from build123d import *

# Parameters (mm, degrees)
SKETCH1_W                 = 50.8889
SKETCH1_H                 = 6.35
BOSS_EXTRUDE1_DEPTH       = 225.99904
SKETCH3_R                 = 5.000000033
CUT_EXTRUDE1_DEPTH        = 228.515512914
LPATTERN1_COUNT           = 3
LPATTERN1_PITCH           = 11.500000114
LPATTERN1_COUNT_DIR2      = 3
LPATTERN1_PITCH_DIR2      = 11.500000114
LPATTERN2_COUNT           = 2
LPATTERN2_PITCH           = 66.00000008
LPATTERN2_COPY_1_SKETCH_R = 5.000000033
LPATTERN2_COPY_1_DEPTH    = 228.515512914
LPATTERN2_COPY_2_SKETCH_R = 5.000000033
LPATTERN2_COPY_2_DEPTH    = 228.515512914
LPATTERN2_COPY_3_SKETCH_R = 5.000000033
LPATTERN2_COPY_3_DEPTH    = 228.515512914
LPATTERN2_COPY_4_SKETCH_R = 5.000000033
LPATTERN2_COPY_4_DEPTH    = 228.515512914
LPATTERN2_COPY_5_SKETCH_R = 5.000000033
LPATTERN2_COPY_5_DEPTH    = 228.515512914
LPATTERN2_COPY_6_SKETCH_R = 5.000000033
LPATTERN2_COPY_6_DEPTH    = 228.515512914
LPATTERN2_COPY_7_SKETCH_R = 5.000000033
LPATTERN2_COPY_7_DEPTH    = 228.515512914
LPATTERN2_COPY_8_SKETCH_R = 5.000000033
LPATTERN2_COPY_8_DEPTH    = 228.515512914


with BuildPart() as part:
    # Sketch1 → Boss-Extrude1 (new body)
    with BuildSketch(Plane.XY):
        Rectangle(SKETCH1_W, SKETCH1_H)
    extrude(amount=BOSS_EXTRUDE1_DEPTH)

    # Sketch3 → Cut-Extrude1 (cut, through all)
    with BuildSketch(Plane(origin=(0, 3.175, 0), x_dir=(1, 0, 0), z_dir=(0, 1, 0))):
        with Locations(Location((8.669450022, -180.875882939, 0), (0, 0, 270))):
            Circle(SKETCH3_R)
    cut_extrude1 = extrude(amount=-CUT_EXTRUDE1_DEPTH, mode=Mode.SUBTRACT)

    # LPattern1: Cut-Extrude1 3 × 3
    with Locations(*[(-i * LPATTERN1_PITCH, 0, -j * LPATTERN1_PITCH_DIR2) for i in range(LPATTERN1_COUNT) for j in range(LPATTERN1_COUNT_DIR2) if (i, j) != (0, 0)]):
        add(cut_extrude1, mode=Mode.SUBTRACT)

    # LPattern2: Cut-Extrude1 ×2
    with Locations(*[(0, 0, -i * LPATTERN2_PITCH) for i in range(1, LPATTERN2_COUNT)]):
        add(cut_extrude1, mode=Mode.SUBTRACT)

    # LPattern2 copy 1 sketch → LPattern2 copy 1 (cut, through all)
    with BuildSketch(Plane(origin=(0, 3.175, -77.500000194), x_dir=(1, 0, 0), z_dir=(0, 1, 0))):
        with Locations(Location((8.669450022, -180.875882939, 0), (0, 0, 270))):
            Circle(LPATTERN2_COPY_1_SKETCH_R)
    extrude(amount=-LPATTERN2_COPY_1_DEPTH, mode=Mode.SUBTRACT)

    # LPattern2 copy 2 sketch → LPattern2 copy 2 (cut, through all)
    with BuildSketch(Plane(origin=(0, 3.175, -89.000000308), x_dir=(1, 0, 0), z_dir=(0, 1, 0))):
        with Locations(Location((8.669450022, -180.875882939, 0), (0, 0, 270))):
            Circle(LPATTERN2_COPY_2_SKETCH_R)
    extrude(amount=-LPATTERN2_COPY_2_DEPTH, mode=Mode.SUBTRACT)

    # LPattern2 copy 3 sketch → LPattern2 copy 3 (cut, through all)
    with BuildSketch(Plane(origin=(-11.500000114, 3.175, -66.00000008), x_dir=(1, 0, 0), z_dir=(0, 1, 0))):
        with Locations(Location((8.669450022, -180.875882939, 0), (0, 0, 270))):
            Circle(LPATTERN2_COPY_3_SKETCH_R)
    extrude(amount=-LPATTERN2_COPY_3_DEPTH, mode=Mode.SUBTRACT)

    # LPattern2 copy 4 sketch → LPattern2 copy 4 (cut, through all)
    with BuildSketch(Plane(origin=(-11.500000114, 3.175, -77.500000194), x_dir=(1, 0, 0), z_dir=(0, 1, 0))):
        with Locations(Location((8.669450022, -180.875882939, 0), (0, 0, 270))):
            Circle(LPATTERN2_COPY_4_SKETCH_R)
    extrude(amount=-LPATTERN2_COPY_4_DEPTH, mode=Mode.SUBTRACT)

    # LPattern2 copy 5 sketch → LPattern2 copy 5 (cut, through all)
    with BuildSketch(Plane(origin=(-11.500000114, 3.175, -89.000000308), x_dir=(1, 0, 0), z_dir=(0, 1, 0))):
        with Locations(Location((8.669450022, -180.875882939, 0), (0, 0, 270))):
            Circle(LPATTERN2_COPY_5_SKETCH_R)
    extrude(amount=-LPATTERN2_COPY_5_DEPTH, mode=Mode.SUBTRACT)

    # LPattern2 copy 6 sketch → LPattern2 copy 6 (cut, through all)
    with BuildSketch(Plane(origin=(-23.000000228, 3.175, -66.00000008), x_dir=(1, 0, 0), z_dir=(0, 1, 0))):
        with Locations(Location((8.669450022, -180.875882939, 0), (0, 0, 270))):
            Circle(LPATTERN2_COPY_6_SKETCH_R)
    extrude(amount=-LPATTERN2_COPY_6_DEPTH, mode=Mode.SUBTRACT)

    # LPattern2 copy 7 sketch → LPattern2 copy 7 (cut, through all)
    with BuildSketch(Plane(origin=(-23.000000228, 3.175, -77.500000194), x_dir=(1, 0, 0), z_dir=(0, 1, 0))):
        with Locations(Location((8.669450022, -180.875882939, 0), (0, 0, 270))):
            Circle(LPATTERN2_COPY_7_SKETCH_R)
    extrude(amount=-LPATTERN2_COPY_7_DEPTH, mode=Mode.SUBTRACT)

    # LPattern2 copy 8 sketch → LPattern2 copy 8 (cut, through all)
    with BuildSketch(Plane(origin=(-23.000000228, 3.175, -89.000000308), x_dir=(1, 0, 0), z_dir=(0, 1, 0))):
        with Locations(Location((8.669450022, -180.875882939, 0), (0, 0, 270))):
            Circle(LPATTERN2_COPY_8_SKETCH_R)
    extrude(amount=-LPATTERN2_COPY_8_DEPTH, mode=Mode.SUBTRACT)


solid = part.part
Design review of the part built by this model. Coordinates are the model's own, in mm. Give positions to 0.01 mm unless a question says otherwise; leave off trailing zeros. Write each loop counter-clockwise with the first axis right and the second up, starting at its lowest first coordinate (ties: lowest second). Pieces come first, ordered by that corner, then holes. Notation, with made-up numbers: M -20.75,-30.75 L 10.25,-30.75 A20 cw 10.25,-4.75 Z; hole C 56,84 d1. An arc over 180 degrees is marked long. Return JSON: item names as keys, results as strings. Group by question number.
Item 1: Take a section at B-B (x = 11). Give the boundary of the cut face in (y, z) (3 decimals), plus the area to 3 significant figures.
Item 2: Wall thickness on line 1 along X through (y, z) = (-2.5, 158); line 2 along X through (y, z) = (1, 93.5): over which ranges is each line inside the solid? List them lowest first.
Item 3: Take a section at C-C (y = -1.75). Count the separate pieces of the cut face and the enclosed holes in it, plus the area to 3 significant figures.
Item 4: Take a section at A-A (z = 89). Give the boundary of the cut face in (x, y) (3 decimals), plus the area to 3 significant figures.
Item 5: Clearance check with a flat-ended pin moving along its axis: pin 1 Ø6 at (x, z) = (8.67, 180.88) entering from -Y. State where the tip first meets the part, or that it passes through.
Item 6: The part is to be moulded in two halves that separate along X. For faces 1 (the cylindrical face through (-4.746, 0.044, 173.995)), 2 (the flat face through (25.444, 0, 111)), 3 (the flat face through (17, 3.175, 111)), 4 (the cylindrical face through (-14.11, 0.04, 109.88)), say which applies: pulls with the +X half, pulls with the -X half, needs draft (parallel to the pull), parting line crosses it, or undercut.
Item 7: Take a section at D-D (x = -5.5). Give the boundary of the cut face in (y, z) (3 decimals).
Return value:
{
 "1": {"outline": "M -3.175,0 L 3.175,0 L 3.175,87.452 L -3.175,87.452 Z; M -3.175,96.3 L 3.175,96.3 L 3.175,98.952 L -3.175,98.952 Z; M -3.175,107.8 L 3.175,107.8 L 3.175,110.452 L -3.175,110.452 Z; M -3.175,119.3 L 3.175,119.3 L 3.175,153.452 L -3.175,153.452 Z; M -3.175,162.3 L 3.175,162.3 L 3.175,164.952 L -3.175,164.952 Z; M -3.175,173.8 L 3.175,173.8 L 3.175,176.452 L -3.175,176.452 Z; M -3.175,185.3 L 3.175,185.3 L 3.175,225.999 L -3.175,225.999 Z", "area": "1,100 mm2"},
 "2": {"line 1": "x = -25.44 to -19.33, -9.33 to -7.83, 2.17 to 3.67, 13.67 to 25.44", "line 2": "x = -25.44 to -19.06, -9.6 to -7.56, 1.9 to 3.94, 13.4 to 25.44"},
 "3": {"separate pieces": "1", "enclosed holes": "18", "area": "10,100 mm2"},
 "4": {"outline": "M -25.444,-3.175 L -18.421,-3.175 L -18.421,3.175 L -25.444,3.175 Z; M -10.24,-3.175 L -6.921,-3.175 L -6.921,3.175 L -10.24,3.175 Z; M 1.26,-3.175 L 4.579,-3.175 L 4.579,3.175 L 1.26,3.175 Z; M 12.76,-3.175 L 25.444,-3.175 L 25.444,3.175 L 12.76,3.175 Z", "area": "167 mm2"},
 "5": {"pin 1": "passes through"},
 "6": {"face 1": "undercut", "face 2": "pulls with the +X half", "face 3": "needs draft", "face 4": "undercut"},
 "7": {"outline": "M -3.175,0 L 3.175,0 L 3.175,87.648 L -3.175,87.648 Z; M -3.175,96.104 L 3.175,96.104 L 3.175,99.148 L -3.175,99.148 Z; M -3.175,107.604 L 3.175,107.604 L 3.175,110.648 L -3.175,110.648 Z; M -3.175,119.104 L 3.175,119.104 L 3.175,153.648 L -3.175,153.648 Z; M -3.175,162.104 L 3.175,162.104 L 3.175,165.148 L -3.175,165.148 Z; M -3.175,173.604 L 3.175,173.604 L 3.175,176.648 L -3.175,176.648 Z; M -3.175,185.104 L 3.175,185.104 L 3.175,225.999 L -3.175,225.999 Z"}
}
